Can you work these out from the model? Positions are in its coordinate system, mm. Face numbers are marked on the shaded views. A direction names the side the tool comes from. Give positions to 0.01 mm unless a question says otherwise; leave off trailing zeros. Write each loop counter-clockwise with the first axis right and the second up, starting at its lowest first coordinate (ties: lowest second). Pieces come first, ordered by that corner, then holes. Notation, with made-up numbers: M 37.5,8 L 88.5,8 A31 ccw 88.5,42 Z; hole C 10.25,79 d6. An arc over 180 degrees is marked long. Answer as CSV lines item,"result". Start each with the question number.
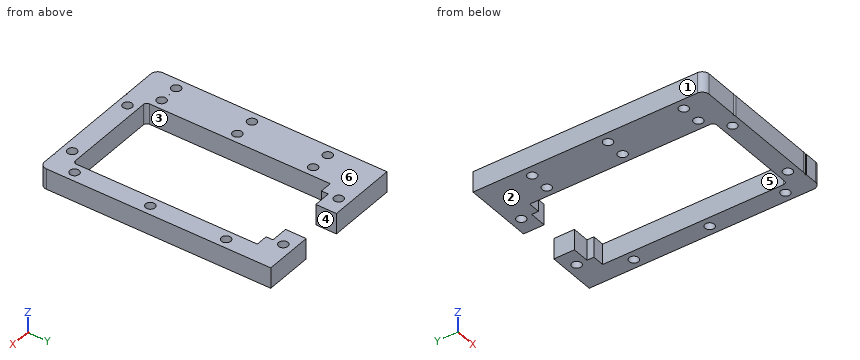
Autodesk Inventor part; units mm, degrees
ref_plane "YZ Plane" through (0, 0, 0) normal (1, 0, 0) x (0, 1, 0)
ref_plane "XZ Plane" through (0, 0, 0) normal (0, 1, 0) x (-1, 0, 0)
ref_plane "XY Plane" through (0, 0, 0) normal (0, 0, 1) x (1, 0, 0)
ref_plane "작업 평면1" through (0, 0, 0) normal (0, 0, 1) x (1, 0, 0)
sketch "스케치1" plane through (0, 0, 0) normal (0, 0, 1) x (1, 0, 0)
  arc A0 (20.1, 4.5766) -> (19.5808, 6.2636) centre (17.1, 4.5766) ccw
  line L0 (19.5808, 6.2636) -> (15.5953, 12.1246)
  arc A1 (15.5953, 12.1246) -> (13.9414, 13) centre (13.9414, 11) ccw
  line L1 (13, 13) -> (13.9414, 13)
  arc A2 (14.5, 11.5) -> (13, 13) centre (13, 11.5) ccw
  line L2 (14.5, -41.5) -> (14.5, 11.5)
  arc A3 (13.5, -42.5) -> (14.5, -41.5) centre (13.5, -41.5) ccw
  line L3 (-13.5, -42.5) -> (13.5, -42.5)
  arc A4 (-14.5, -41.5) -> (-13.5, -42.5) centre (-13.5, -41.5) ccw
  line L4 (-14.5, 11.5) -> (-14.5, -41.5)
  arc A5 (-13, 13) -> (-14.5, 11.5) centre (-13, 11.5) ccw
  line L5 (-13.9414, 13) -> (-13, 13)
  arc A6 (-13.9414, 13) -> (-15.5953, 12.1246) centre (-13.9414, 11) ccw
  line L6 (-15.5953, 12.1246) -> (-19.5808, 6.2636)
  arc A7 (-19.5808, 6.2636) -> (-20.1, 4.5766) centre (-17.1, 4.5766) ccw
  line L7 (-20.1, 4.5766) -> (-20.1, -39.6766)
  arc A8 (-20.1, -39.6766) -> (-19.5808, -41.3636) centre (-17.1, -39.6766) ccw
  line L8 (-19.5808, -41.3636) -> (-15.8929, -46.7869)
  arc A9 (-15.8929, -46.7869) -> (-13.4121, -48.1) centre (-13.4121, -45.1) ccw
  line L9 (-13.4121, -48.1) -> (13.4121, -48.1)
  arc A10 (13.4121, -48.1) -> (15.8929, -46.7869) centre (13.4121, -45.1) ccw
  line L10 (15.8929, -46.7869) -> (19.5808, -41.3636)
  arc A11 (19.5808, -41.3636) -> (20.1, -39.6766) centre (17.1, -39.6766) ccw
  line L11 (20.1, -39.6766) -> (20.1, 4.5766)
  circle A12 centre (-17.3, 4) radius 1.35
  circle A13 centre (-17.3, -18) radius 1.35
  circle A14 centre (-11, -45.3) radius 1.35
  circle A15 centre (17.3, 4) radius 1.35
  circle A16 centre (17.3, -18) radius 1.35
  circle A17 centre (11, -45.3) radius 1.35
  circle A18 centre (-17.3, -40) radius 1.35
  circle A19 centre (17.3, -40) radius 1.35
  line L12 (-20.1, -48.0993) -> (-20.1, 25.0993)
  line L13 (-20.1, 25.0993) -> (-26.1, 25.0993)
  line L14 (-26.1, -48.0993) -> (-26.1, 25.0993)
  line L15 (-20.1, -48.0993) -> (-26.1, -48.0993)
  line L16 (-14.5, 11.5) -> (-14.5, 13.7353)
  line L17 (-13.9414, 13) -> (-15.2676, 13)
  line L18 (-14.5, -41.5) -> (-14.5, -54.5935)
  line L19 (-20.1, -48.0993) -> (-13.475, -48.0993)
  line L20 (-13.475, -48.0993) -> (-26.1, -48.0993)
  line L21 (-26.1, -48.0993) -> (-26.1, 13)
  line L22 (-26.1, 13) -> (-13.475, 13)
  line L23 (-13.475, 13) -> (-13.475, -48.0993)
  line L24 (-17.3, 4) -> (-17.3, -18)
  line L25 (-17.3, -18) -> (-23.1, -18)
  line L26 (-23.1, -18) -> (-23.1, 4)
  line L27 (-23.1, 4) -> (-17.3, 4)
  line L28 (-17.3, -18) -> (-17.3, -40)
  line L29 (-17.3, -40) -> (-23.1, -40)
  line L30 (-23.1, -40) -> (-23.1, -18)
  line L31 (-23.1, -18) -> (-17.3, -18)
  circle A20 centre (-23.1, 4) radius 1.35
  circle A21 centre (-23.1, -18) radius 1.35
  circle A22 centre (-23.1, -40) radius 1.35
  line L32 (14.5, 13) -> (14.5, -48.0993)
  line L33 (14.5, -48.0993) -> (20.1, -48.0993)
  line L34 (20.1, -48.0993) -> (20.1, 13)
  line L35 (20.1, 13) -> (14.5, 13)
  circle A23 centre (-23.1, 4) radius 1.35
  circle A24 centre (-23.1, -18) radius 1.35
  circle A25 centre (-23.1, -40) radius 1.35
  point P0 (0, 0)
  point P1 (-14.5, 13)
  point P2 (20.1, 4.5766)
  point P3 (14.5, 11.5)
  point P4 (-26.1, 13)
  point P5 (-14.5, -48.0993)
  point P6 (-14.5, -47.8958)
  point P7 (14.5, -47.8958)
  point P8 (20.1, -39.6766)
  point P9 (-20.0825, -40)
  point P10 (-20.1, -40)
  dimension "d0" = 2.7
  dimension "d1" = 2.7
  dimension "d2" = 2.7
extrude "돌출1" add sketch "스케치1" along normal blind 6 contours L11 A11 L10 A10 L32 L2 A1 L0 A0 | A0 L0 A1 L32 L35 L34 | L34 L33 L32 A10 L10 A11 | A10 L9 A9 L23 L3 A3 L32 | L23 A9 L18 A4 L3 | L18 L19 L12 L29 A8 L8 A9 | A9 L8 A8 L29 A18 L28 A13 L24 A12 L27 L7 A7 L6 A6 L16 L4 L18 | L15 L14 L22 L12 L7 L27 A20 L26 A21 L30 A22 L29 | A6 L6 A7 L12 L22 L17 L16 | L29 A22 L30 A21 L25 L7 L12 | A8 L7 L25 A13 L28 A18 L29 | L25 A21 L26 A20 L27 L7 | L7 L27 A12 L24 A13 L25
fillet "모깎기1" radius 2 6 edges at (-26.1, -48.0993, 3) (20.1, -48.0993, 3) (20.1, 13, 3) (14.5, 13, 3) (-14.5, 13, 3) (-26.1, 13, 3)
sketch "스케치2" plane through (0, 0, 6) normal (0, 0, 1) x (1, 0, 0)
  line L0 (-13, 13) -> (-13, 19)
  line L1 (13, 13) -> (-13, 13)
  line L2 (13, 13) -> (13, 19)
  line L3 (-13, 19) -> (13, 19)
  arc A0 (-24.1, 13) -> (-26.1, 11) centre (-24.1, 11) ccw
  line L4 (-26.1, 11) -> (-26.1, -46.0993)
  arc A1 (-26.1, -46.0993) -> (-24.1, -48.0993) centre (-24.1, -46.0993) ccw
  line L5 (-24.1, -48.0993) -> (-14.5, -48.0993)
  line L6 (-14.5, -48.0993) -> (-14.5, -47.8958)
  arc A2 (-14.5, -47.8958) -> (-13.4121, -48.1) centre (-13.4121, -45.1) ccw
  line L7 (-13.4121, -48.1) -> (13.4121, -48.1)
  arc A3 (13.4121, -48.1) -> (14.5, -47.8958) centre (13.4121, -45.1) ccw
  line L8 (14.5, -47.8958) -> (14.5, -48.0993)
  line L9 (14.5, -48.0993) -> (18.1, -48.0993)
  arc A4 (18.1, -48.0993) -> (20.1, -46.0993) centre (18.1, -46.0993) ccw
  line L10 (20.1, -46.0993) -> (20.1, 11)
  arc A5 (20.1, 11) -> (18.1, 13) centre (18.1, 11) ccw
  line L11 (18.1, 13) -> (16.5, 13)
  arc A6 (16.5, 13) -> (14.5, 11) centre (16.5, 11) ccw
  line L12 (14.5, 11) -> (14.5, -41.5)
  arc A7 (13.5, -42.5) -> (14.5, -41.5) centre (13.5, -41.5) ccw
  line L13 (13.5, -42.5) -> (-13.5, -42.5)
  arc A8 (-14.5, -41.5) -> (-13.5, -42.5) centre (-13.5, -41.5) ccw
  line L14 (-14.5, -41.5) -> (-14.5, 11)
  arc A9 (-14.5, 11) -> (-16.5, 13) centre (-16.5, 11) ccw
  line L15 (-16.5, 13) -> (-24.1, 13)
  circle A10 centre (-17.3, -18) radius 1.35
  circle A11 centre (-23.1, 4) radius 1.35
  circle A12 centre (-23.1, -18) radius 1.35
  circle A13 centre (11, -45.3) radius 1.35
  circle A14 centre (-11, -45.3) radius 1.35
  circle A15 centre (-17.3, 4) radius 1.35
  circle A16 centre (-17.3, -40) radius 1.35
  circle A17 centre (17.3, -18) radius 1.35
  circle A18 centre (17.3, 4) radius 1.35
  circle A19 centre (17.3, -40) radius 1.35
  arc A20 (-20.1, -39.6766) -> (-20.0825, -40) centre (-17.1, -39.6766) ccw
  line L16 (-20.0825, -40) -> (-20.1, -40)
  line L17 (-20.1, -40) -> (-20.1, -39.6766)
  circle A21 centre (-23.1, -40) radius 1.35
  line L18 (18.1, 11) -> (-24.1, 11)
  line L19 (-24.1, 11) -> (-26.1, 11)
  line L20 (18.1, 11) -> (20.1, 11)
  line L21 (20.1, 11) -> (-26.1, 11)
  line L22 (-26.1, 11) -> (-26.1, 19)
  line L23 (-26.1, 19) -> (20.1, 19)
  line L24 (20.1, 19) -> (20.1, 11)
  line L25 (11, -45.3) -> (-11, -45.3)
  line L26 (-11, -45.3) -> (-11, 16)
  line L27 (-11, 16) -> (11, 16)
  line L28 (11, 16) -> (11, -45.3)
  circle A22 centre (11, 16) radius 1.35
  circle A23 centre (-11, 16) radius 1.35
  line L29 (11, 16) -> (6, 16)
  line L30 (-11, 16) -> (-6, 16)
  line L31 (6, 13) -> (6, 19)
  line L32 (6, 19) -> (-6, 19)
  line L33 (-6, 19) -> (-6, 13)
  line L34 (-6, 13) -> (6, 13)
  point P0 (0, 0)
  point P1 (11, 13)
  point P2 (11, 11)
  point P3 (-11, 13)
  point P4 (-14.5, 11)
  point P5 (-11, 11)
  dimension "d6" = 2.7
  dimension "d7" = 2.7
  dimension "d8" = 5
  dimension "d9" = 5
extrude "돌출2" add sketch "스케치2" against normal blind 6 contours L1 L26 L18 A9 L15 A0 L22 L23 L0 | L0 L3 L33 L27 A23 L26 L1 | L26 A23 L27 L33 L1 | L3 L2 L1 L28 A22 L27 L31 | L31 L27 A22 L28 L1 | L28 L1 L2 L23 L24 A5 L11 A6 L18
properties part number "_body_side_ver2" material "PMMA 플라스틱"
1) On a 3-axis mill with a long thin cutter (end or side, diameter ignored), from which of +Z, -Z, +X, -X, +Y, -Y can I reach the whole of each face in a straight line? I mean the marked faces 4, 5 and 6. Say none if no direction works.
2) I want a section at B-B, the plane y = -32.5. Please give me the cut outline in (x, z).
3) I want a section at C-C, the plane x = -17.3. Please give me the cut outline in (y, z), then the cut area to 3 significant figures.
4) I need wall thicknesses on L1, parallel to Y at x = 17.3, z = 4.3; L2, parallel to X at y = 6, z = 1.4; L3, parallel to Y at x = -10.5, z = 5.1. Which ranges of each line are inside material? Lowest first, please. Write a range as from..to.
5) I want a section at A-A, the plane x = 7. Please give me the cut outline in (y, z).
6) Thinking about a two-plate mould opening in X: for the marked faces 1, 2 and 3, which applies, released by +X, released by -X, zero draft, split by the parting line, or undercut?
7) I want a section at D-D, the plane z = 2.6. State how many separate pieces and enclosed holes the cut face has, then the cut area to 3 significant figures.
Values found:
1,face 4,"+Z, -Z, +Y"
1,face 5,"+Z, -Z"
1,face 6,"+Z, +X, -X, +Y, -Y"
2,outline,"M -26.1,0 L -14.5,0 L -14.5,6 L -26.1,6 Z; M 14.5,0 L 20.1,0 L 20.1,6 L 14.5,6 Z"
3,outline,"M -48.1,0 L -41.35,0 L -41.35,6 L -48.1,6 Z; M -38.65,0 L -19.35,0 L -19.35,6 L -38.65,6 Z; M -16.65,0 L 2.65,0 L 2.65,6 L -16.65,6 Z; M 5.35,0 L 19,0 L 19,6 L 5.35,6 Z"
3,area,"354 mm²"
4,L1,"y = -48.1..-41.35, -38.65..-19.35, -16.65..2.65, 5.35..19"
4,L2,"x = -26.1..-14.5, 14.5..20.1"
4,L3,"y = -48.1..-46.55, -44.05..-42.5, 13..14.75, 17.25..19"
5,outline,"M -48.1,0 L -42.5,0 L -42.5,6 L -48.1,6 Z; M 13,0 L 19,0 L 19,6 L 13,6 Z"
6,face 1,"released by -X"
6,face 2,"zero draft"
6,face 3,"undercut"
7,separate pieces,"1"
7,enclosed holes,"14"
7,area,"1,360 mm²"
